Read the model definition and answer for the solid it produces. Units are mm, in the model's axes. Face numbers are marked on the shaded views. A direction names the side the tool comes from. Give positions to 0.01 mm unless a question says otherwise; leave off trailing zeros. Order: outer loops, then holes, each group sorted by start corner. A loop starts at its lowest first (then second) coordinate and runs counter-clockwise, first axis right, second up. Notation, with made-up numbers: (61, 83.5) - (74, 83.5) arc R6 cw to (74, 92.5) - close; hole circle Ø8 at (70.5, 66). An arc over 180 degrees is marked (long way). Use a Markdown table: item, result. Add a question column.
1. Which of the six approach directions +Z, -Z, +X, -X, +Y, -Y give full straight-line access (tool end or side, diameter ignored) to the marked faces 4 and 5?
2. Consider L1, parallel to X at y = 18, z = -28; L2, parallel to Z at x = 11, y = 2.75; L3, parallel to X at y = 20, z = -66. Determine where each line is inside the solid, lowest interval first.
3. For a pull along X with two mould halves and no side action, classify the marked faces 1, 2 and 3 as released by +X, released by -X, zero draft, split by the parting line, or undercut.
4. A cutting plane is placed at B-B on x = 10.5. Determine the outline of the cut face in (y, z).
5. Flat-ended cylindrical pins translate along their axes: P1, Ø2, axis at x = 38.5, y = 18.5, coming from the +Z side; P2, Ø3.5, axis at x = 36.5, z = -45.5, coming from the -Y side; P3, Ø15, axis at x = 10, z = -57.5, coming from the +Y side. Find the tip coordinate at first contact, or state that the pin passes through.
6. A cutting plane is placed at C-C on z = -65.5. Determine the outline of the cut face in (x, y).
7. A cutting plane is placed at D-D on z = -40. Determine the outline of the cut face in (x, y).
8. A cutting plane is placed at A-A on y = 5. Determine the outline of the cut face in (x, z), and give its area (3 significant figures).
Autodesk Inventor part; units mm, degrees
ref_plane "YZ Plane" through (0, 0, 0) normal (1, 0, 0) x (0, 1, 0)
ref_plane "XZ Plane" through (0, 0, 0) normal (0, 1, 0) x (-1, 0, 0)
ref_plane "XY Plane" through (0, 0, 0) normal (0, 0, 1) x (1, 0, 0)
sketch "Náčrt1" plane through (0, 0, 0) normal (0, 1, 0) x (-1, 0, 0)
  line L0 (0, 0) -> (-30, 0)
  line L1 (-30, 0) -> (-30, -80)
  line L2 (-30, -80) -> (0, -80)
  line L3 (0, -80) -> (0, 0)
  line L4 (2.5, 2.5) -> (-32.5, 2.5)
  line L5 (-32.5, 2.5) -> (-32.5, -82.5)
  line L6 (-32.5, -82.5) -> (2.5, -82.5)
  line L7 (2.5, -82.5) -> (2.5, 2.5)
  dimension "d0" = 80
  dimension "d1" = 30
  dimension "d2" = 2.5
extrude "Vysunutí1" add sketch "Náčrt1" along normal blind 2 contours L3 L2 L1 L0
extrude "Vysunutí2" add sketch "Náčrt1" along normal blind 22
sketch "Náčrt2" plane through (32.5, 0, 2.5) normal (1, 0, 0) x (0, 0, -1)
  line L0 (0, 22) -> (85, 22)
  line L1 (30, 22) -> (55, 22)
  line L2 (55, 22) -> (55, 20)
  line L3 (55, 20) -> (30, 20)
  line L4 (30, 20) -> (30, 22)
  line L5 (85, 0) -> (85, 22)
  line L6 (0, 0) -> (0, 22)
  point P0 (2.5, 0)
  dimension "d7" = 30
  dimension "d8" = 30
  dimension "d9" = 2
extrude "Vysunutí3" add sketch "Náčrt2" along normal blind 8.8
sketch "Náčrt3" plane through (32.5, 20, -52.5) normal (0, -1, 0) x (1, 0, 0)
  line L0 (0, 25) -> (8.8, 25)
  line L1 (0, 0) -> (8.8, 0)
  line L2 (8.8, 25) -> (6.8, 25)
  line L3 (6.8, 25) -> (6.8, 0)
  line L4 (6.8, 0) -> (8.8, 0)
  line L5 (8.8, 0) -> (8.8, 25)
  point P0 (-32.5, 52.5)
  point P1 (8.8, 0)
  point P2 (6.8, 25)
  dimension "d12" = 2
extrude "Vysunutí4" add sketch "Náčrt3" along normal blind 6
fillet "Zaoblení1" radius 2 3 edges at (41.3, 22, -40) (32.5, 21, -52.5) (32.5, 21, -27.5)
fillet "Zaoblení2" radius 2 4 edges at (-2.5, 11, 2.5) (32.5, 11, 2.5) (32.5, 11, -82.5) (-2.5, 11, -82.5)
fillet "Zaoblení3" radius 2 4 edges at (30, 12, -80) (30, 12, 0) (0, 12, -80) (0, 12, 0)
equation "\"d8\" = d7"
properties part number "AccesoryHolder"
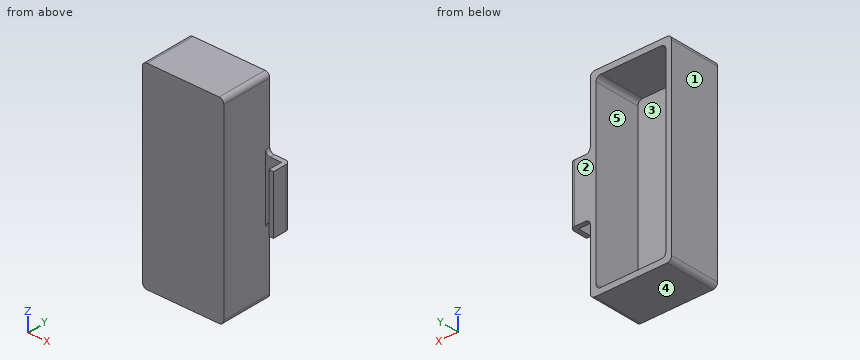
Output values:
| question | item | result |
|---|---|---|
| 1 | face 4 | -Z, +X, -X, +Y, -Y |
| 1 | face 5 | +Y |
| 2 | L1 | -2.5 to 0, 30 to 32.5, 39.3 to 41.3 |
| 2 | L2 | -82.5 to -80, 0 to 2.5 |
| 2 | L3 | -2.5 to 0, 30 to 32.5 |
| 3 | face 1 | released by -X |
| 3 | face 2 | zero draft |
| 3 | face 3 | undercut |
| 4 | outline | (0, -82.5) - (22, -82.5) - (22, -80) - (2, -80) - (2, 0) - (22, 0) - (22, 2.5) - (0, 2.5) - close |
| 5 | P1 | z = -27.5 |
| 5 | P2 | y = 20 |
| 5 | P3 | y = 2 |
| 6 | outline | (-2.5, 0) - (32.5, 0) - (32.5, 22) - (30, 22) - (30, 2) - (0, 2) - (0, 22) - (-2.5, 22) - close |
| 7 | outline | (-2.5, 0) - (32.5, 0) - (32.5, 20) - (39.3, 20) - (39.3, 14) - (41.3, 14) - (41.3, 20) arc R2 ccw to (39.3, 22) - (30, 22) - (30, 2) - (0, 2) - (0, 22) - (-2.5, 22) - close |
| 8 | outline | (-2.5, -80.5) arc R2 ccw to (-0.5, -82.5) - (30.5, -82.5) arc R2 ccw to (32.5, -80.5) - (32.5, 0.5) arc R2 ccw to (30.5, 2.5) - (-0.5, 2.5) arc R2 ccw to (-2.5, 0.5) - close; hole (0, -78) arc R2 ccw to (2, -80) - (28, -80) arc R2 ccw to (30, -78) - (30, -2) arc R2 ccw to (28, 0) - (2, 0) arc R2 ccw to (0, -2) - close |
| 8 | area | 575 mm² |
